Source: CAD feature listing. Evaluate the final solid. Frame: model axes, mm. A direction names the side the tool comes from. Round coordinates to 2 decimals unless told otherwise and drop trailing zeros. Write each loop counter-clockwise with the first axis right and the second up, starting at its lowest first coordinate (ties: lowest second). Pieces come first, ordered by that corner, then holes. Notation, with made-up numbers: (15, -32) -> (74, -32) arc R24 ccw to (74, -1) -> close; hole circle Ø11 at (44.5, -28.5). An arc over 180 degrees is marked (long way). Put each result on its own line as item: value.
```python
from build123d import *

# Parameters (mm, degrees)
F1_DEPTH = 76.2
F3_DEPTH = 25.4
F4_R     = 7.797698
F5_DEPTH = 127


with BuildPart() as f1:
    # F0 (on Front) → F1 (new body)
    with BuildSketch(Plane.XZ):
        Polygon((-50.381906, 0), (0, 0), (25.614025, 0), (-17.3402, 68.811595), (-50.381906, 68.811595), align=None)
    extrude(amount=F1_DEPTH)

    # F2 (on Front) → F3 (join)
    with BuildSketch(Plane.XZ):
        Polygon((-50.381906, 68.811595), (-50.381906, 0), (33.250909, 0), (-15.932729, 76.084539), (-50.381906, 76.084539), align=None)
    extrude(amount=-F3_DEPTH)

    # F4 (on face) → F5 (cut)
    with BuildSketch(Plane(origin=(-50.381906, 0, 0), x_dir=(0, -1, 0), z_dir=(-1, 0, 0))):
        with Locations((38.1, 30.711595)):
            Circle(F4_R)
    extrude(amount=-F5_DEPTH, mode=Mode.SUBTRACT)


solid = f1.part
```
Q1. Cut plane A-A on y = -38.1. Output: boundary loops of the cut face in (x, z).
Ans:
outline: (-50.38, 0) -> (25.61, 0) -> (11.31, 22.91) -> (-50.38, 22.91) -> close; (-50.38, 38.51) -> (1.58, 38.51) -> (-17.34, 68.81) -> (-50.38, 68.81) -> close
Q2. Material intervals for line 1 (Z direction, x = -36, y = -38); line 2 (Z direction, x = -37.5, y = -63.5); line 3 (Y direction, x = -45, z = 25), sorted ascending. Write a range as [from, to].
Ans:
line 1: z = [0, 22.91], [38.51, 68.81]
line 2: z = [0, 68.81]
line 3: y = [-76.2, -43.41], [-32.79, 25.4]
Q3. Cut plane C-C on x = -10. Output: boundary loops of the cut face in (y, z), and give its area (3 significant figures).
Ans:
outline: (-76.2, 0) -> (25.4, 0) -> (25.4, 66.91) -> (0, 66.91) -> (0, 57.05) -> (-76.2, 57.05) -> close; hole circle Ø15.6 at (-38.1, 30.71)
area: 5,860 mm^2
Q4. Draft query along Z for faces 1 (the flat face through (-9, -26, 0)), 2 (the cylindrical face through (-19.9, -36.4, 23.1)), 3 (the flat face through (-21, -76.2, 27)). Return one class per face: +Z half, -Z half, draft (parallel to the pull), parting line (faces both ways), or undercut.
Ans:
face 1: -Z half
face 2: undercut
face 3: draft
Q5. Pin query (flat end, axial travel): pin 1 (6 mm diameter, centred on x = 2, y = -13.5, fed in from +Z) (3 decimals); pin 2 (1.5 mm diameter, centred on y = -57.5, z = 20, fed in from +X); pin 3 (4 mm diameter, centred on x = -28, y = -16, fed in from -Z); pin 4 (10 mm diameter, centred on y = -28, z = 68, fed in from +X). Return the tip coordinate at first contact, or that it passes through.
Ans:
pin 1: stops at z = 42.635
pin 2: stops at x = 13.6
pin 3: stops at z = 0
pin 4: stops at x = -13.71
Q6. Reachability of faces 4 (the flat face through (-33, 13, 76.085)), 5 (the flat face through (-34, -38, 68.812)), 6 (the flat face through (-6, 0, 52)) from +Z, -Z, +X, -X, +Y, -Y: full face, straight path, thin tool, end or side. Return the list, or none.
Ans:
face 4: +Z, +X, -X, +Y, -Y
face 5: +Z, +X, -X, -Y
face 6: +Z, +X, -Y
Q7. Cut plane D-D on y = -6. Output: boundary loops of the cut face in (x, z), and give its area (3 significant figures).
Ans:
outline: (-50.38, 0) -> (25.61, 0) -> (-17.34, 68.81) -> (-50.38, 68.81) -> close
area: 3,750 mm^2
Q8. Cut plane B-B on z = 29. Output: boundary loops of the cut face in (x, y), and give its area (3 significant figures).
Ans:
outline: (-50.38, -76.2) -> (7.51, -76.2) -> (7.51, -45.71) -> (-50.38, -45.71) -> close; (-50.38, -30.49) -> (7.51, -30.49) -> (7.51, 0) -> (14.5, 0) -> (14.5, 25.4) -> (-50.38, 25.4) -> close
area: 5,180 mm^2
